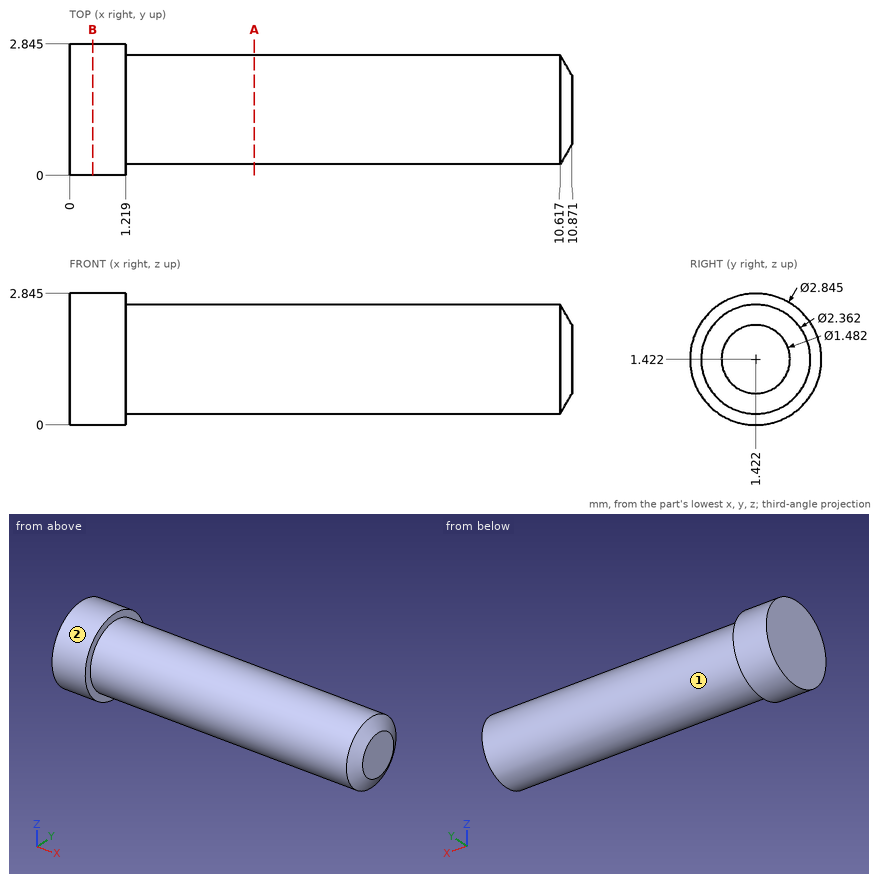
Here's the drawing with two shaded views (mm, measured from the low corner). I have some questions. A direction names the side the tool comes from. Give positions to 0.01 mm unless a question says otherwise; leave off trailing zeros. Write each loop counter-clockwise with the first axis right and the second up, starting at its lowest first coordinate (ties: lowest second). Pieces come first, ordered by that corner, then holes. Notation, with made-up numbers: (80, 5) -> (89, 5) arc R14 cw to (89, 18) -> close; hole circle Ø4 at (11, 69). An arc over 180 degrees is marked (long way). Answer as a JSON object with one key per item and string values. Group by question number.
Item 1: I'm going to push flat-ended pins straight in: P1, Ø1.5, axis at x = 6, z = 1, coming from the -Y side; P2, Ø1, axis at x = 8, z = 2.5, coming from the -Y side. Where does each tip first touch, or does it pass through?
Item 2: Please list where these lines run through material, in increasing order: line 1 (Z direction, x = 5.25, y = 1.5); line 2 (Y direction, x = 10.5, z = 2.4) (1 decimal); line 3 (Y direction, x = 7.5, z = 1.1) (1 decimal). Write a range as [from, to].
Item 3: Suppose I cut it at A-A (x = 4). Please give me the cut outline in (y, z).
Item 4: Suppose I cut it at B-B (x = 0.5). Please give me the cut outline in (y, z) (1 decimal).
Item 5: For the marked faces 1 and 2, which set-ups out of +Z, -Z, +X, -X, +Y, -Y let a thin tool reach every point of the face, with its end or its side?
Findings:
{
 "1": {"P1": "stops at y = 0.24", "P2": "stops at y = 0.39"},
 "2": {"line 1": "z = [0.24, 2.6]", "line 2": "y = [0.8, 2.1]", "line 3": "y = [0.3, 2.6]"},
 "3": {"outline": "circle Ø2.36 at (1.42, 1.42)"},
 "4": {"outline": "circle Ø2.8 at (1.4, 1.4)"},
 "5": {"face 1": "+X", "face 2": "+X, -X"}
}
